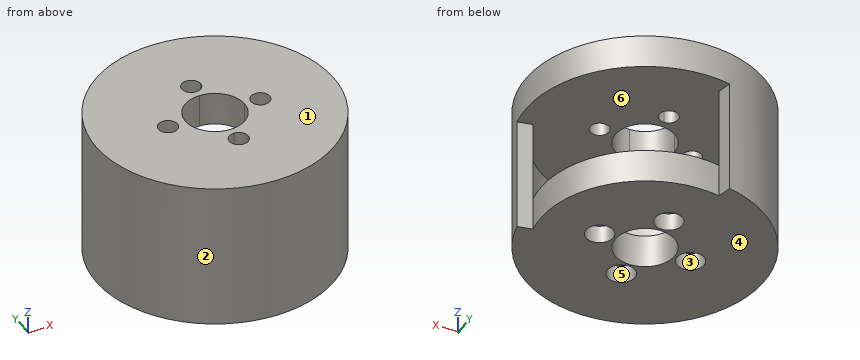
```python
from build123d import *

# Parameters (mm, degrees)
F0_R      = 25.4
F0_R_2    = 22.225
F0_R_3    = 6.35
F1_DEPTH  = 7.112
F2_R      = 25.4
F2_R_2    = 22.225
F3_DEPTH  = 17.272
F4_R      = 2.032
F5_DEPTH  = 21.29049
F6_R      = 2.921
F7_DEPTH  = 3.81
F9_DEPTH  = 17.272
F10_R     = 25.4
F10_R_2   = 2.032
F11_DEPTH = 7.112
F12_DEPTH = 25.4


with BuildPart() as f1:
    # F0 (on Top) → F1 (new body)
    with BuildSketch(Plane.XY):
        with Locations((-2.9115700163, -0.1164628848)):
            Circle(F0_R)
        with Locations((-2.9115700163, -0.1164628848)):
            Circle(F0_R_2, mode=Mode.SUBTRACT)
        with Locations((-2.9115700163, -0.1164628848)):
            Circle(F0_R_2)
        with Locations((-2.9115700163, -0.1164628848)):
            Circle(F0_R_3, mode=Mode.SUBTRACT)
    extrude(amount=F1_DEPTH)

    # F2 (on face) → F3 (join)
    with BuildSketch(Plane.XY.offset(7.112)):
        with Locations((-2.9115700163, -0.1164628848)):
            Circle(F2_R)
        with Locations((-2.9115700163, -0.1164628848)):
            Circle(F2_R_2, mode=Mode.SUBTRACT)
    extrude(amount=F3_DEPTH)

    # F4 (on face) → F5 (cut)
    with BuildSketch(Plane.XY.offset(7.112)):
        with Locations((-2.9115700163, 9.6625371152)):
            Circle(F4_R)
        with Locations((-12.6905700163, -0.1164628848)):
            Circle(F4_R)
        with Locations((6.8674299837, -0.1164628848)):
            Circle(F4_R)
        with Locations((-2.9115700163, -9.8954628848)):
            Circle(F4_R)
    extrude(amount=-F5_DEPTH, mode=Mode.SUBTRACT)

    # F6 (on face) → F7 (cut)
    with BuildSketch(Plane.XY):
        with Locations((-2.9112251941, -9.8947474398)):
            Circle(F6_R)
        with Locations((6.8677748059, -0.1157474398)):
            Circle(F6_R)
        with Locations((-2.9112251941, 9.6632525602)):
            Circle(F6_R)
        with Locations((-12.6902251941, -0.1157474398)):
            Circle(F6_R)
    extrude(amount=F7_DEPTH, mode=Mode.SUBTRACT)

    # F8 (on face) → F9 (cut)
    with BuildSketch(Plane.XY.offset(24.384)):
        with BuildLine():
            ThreePointArc((-7.4796047728, 21.634024086), (12.685813093, 15.5216009657), (18.8507418749, -4.6278269968))
            Line((18.8507418749, -4.6278269968), (21.9596435736, -5.2723075843))
            ThreePointArc((21.9596435736, -5.2723075843), (15.0679881207, 17.9099891283), (-8.1321811666, 24.7412365103))
            Line((-8.1321811666, 24.7412365103), (-7.4796047728, 21.634024086))
        make_face()
    extrude(amount=-F9_DEPTH, mode=Mode.SUBTRACT)

    # F10 (on face) → F11 (join)
    with BuildSketch(Plane.XY.offset(24.384)):
        with Locations((-2.9115700163, -0.1164628848)):
            Circle(F10_R)
        with BuildLine():
            ThreePointArc((-0.8795700163, -9.8954628848), (-4.3484109957, -11.3323038641), (-2.9115700163, -7.8634628848))
            ThreePointArc((-2.9115700163, -7.8634628848), (-1.4747290369, -8.4586219054), (-0.8795700163, -9.8954628848))
        make_face(mode=Mode.SUBTRACT)
        with Locations((-13.0211196663, -0.1164628848)):
            Circle(F10_R_2, mode=Mode.SUBTRACT)
        with BuildLine():
            ThreePointArc((-2.9115700163, 6.2335371152), (1.5785580442, 4.3736651758), (3.4384299837, -0.1164628848))
            ThreePointArc((3.4384299837, -0.1164628848), (1.5785580442, -4.6065909453), (-2.9115700163, -6.4664628848))
            ThreePointArc((-2.9115700163, -6.4664628848), (-7.4016980768, -4.6065909453), (-9.2615700163, -0.1164628848))
            ThreePointArc((-9.2615700163, -0.1164628848), (-7.4016980768, 4.3736651758), (-2.9115700163, 6.2335371152))
        make_face(mode=Mode.SUBTRACT)
        with BuildLine():
            ThreePointArc((8.8994299837, -0.1164628848), (6.8674299837, -2.1484628848), (4.8354299837, -0.1164628848))
            ThreePointArc((4.8354299837, -0.1164628848), (6.8674299837, 1.9155371152), (8.8994299837, -0.1164628848))
        make_face(mode=Mode.SUBTRACT)
        with BuildLine():
            ThreePointArc((-0.8795700163, 9.6625371152), (-1.4747290369, 8.2256961359), (-2.9115700163, 7.6305371152))
            ThreePointArc((-2.9115700163, 7.6305371152), (-4.3484109957, 11.0993780946), (-0.8795700163, 9.6625371152))
        make_face(mode=Mode.SUBTRACT)
    extrude(amount=F11_DEPTH)

    # F8 (on face) → F12 (cut)
    with BuildSketch(Plane.XY.offset(24.384)):
        with BuildLine():
            ThreePointArc((-7.4796047728, 21.634024086), (12.685813093, 15.5216009657), (18.8507418749, -4.6278269968))
            Line((18.8507418749, -4.6278269968), (21.9596435736, -5.2723075843))
            ThreePointArc((21.9596435736, -5.2723075843), (15.0679881207, 17.9099891283), (-8.1321811666, 24.7412365103))
            Line((-8.1321811666, 24.7412365103), (-7.4796047728, 21.634024086))
        make_face()
    extrude(amount=-F12_DEPTH, mode=Mode.SUBTRACT)


solid = f1.part
```
Read the model definition and answer for the solid it produces. Units are mm, in the model's axes. Face numbers are marked on the shaded views. A direction names the side the tool comes from. Give positions to 0.01 mm unless a question says otherwise; leave off trailing zeros. Order: outer loops, then holes, each group sorted by start corner. A loop starts at its lowest first (then second) coordinate and runs counter-clockwise, first axis right, second up.
(1) For a pull along X with two mould halves and no side action, classify the marked faces 1, 2 and 3 as released by +X, released by -X, zero draft, split by the parting line, or undercut.
(2) Find section C-C (x = 1). Give the vertices of the cut face in (y, z).
(3) Find section B-B (z = 29). Give the vertices of the cut face in (x, y).
(4) Given pin 1 (1.5 mm diameter, centred on x = -5.5, z = 21.5, fed in from -Y); pin 2 (5.5 mm diameter, centred on x = 6.87, y = -0.12, fed in from -Z); pin 3 (2 mm diameter, centred on y = 17.5, z = 25, fed in from +X), each flat-ended and moving along its own axis, determine where each tip first touches the part or whether it passes through.
(5) Find section A-A (y = 9). Give the vertices of the cut face in (x, z), plus the area to 3 significant figures.
(6) Straight lines are drawn through the part: L1, parallel to Z at x = 4, y = -14; L2, parallel to Y at x = -1.5, z = 28.5; L3, parallel to Y at x = -3.5, z = 22.5. For each, find the intervals that lie inside material, in ascending order.
(7) Find section D-D (y = -19.5). Give the vertices of the cut face in (x, z), plus the area to 3 significant figures.
(8) For the marked faces 4, 5 and 6, determine the directions among +Z, -Z, +X, -X, +Y, -Y from which every point of the face is accessible in a straight line to the end or side of a thin tool.
Result sheet:
1. face 1: zero draft
1. face 2: split by the parting line
1. face 3: undercut
2. outline: (-25.21, 0) - (-5.12, 0) - (-5.12, 7.11) - (-21.99, 7.11) - (-21.99, 24.38) - (-5.12, 24.38) - (-5.12, 31.5) - (-25.21, 31.5) - close; (4.89, 0) - (21.68, 0) - (21.68, 7.11) - (4.89, 7.11) - close; (4.89, 24.38) - (24.98, 24.38) - (24.98, 31.5) - (4.89, 31.5) - close
3. outline: circle Ø50.8 at (-2.91, -0.12); hole circle Ø4.06 at (-13.02, -0.12); hole circle Ø12.7 at (-2.91, -0.12); hole circle Ø4.06 at (-2.91, -9.9); hole circle Ø4.06 at (-2.91, 9.66); hole circle Ø4.06 at (6.87, -0.12)
4. pin 1: stops at y = -25.45
4. pin 2: stops at z = 3.81
4. pin 3: stops at x = 16.3
5. outline: (-26.62, 0) - (-5.76, 0) - (-5.76, 3.81) - (-4.83, 3.81) - (-4.83, 7.11) - (-23.18, 7.11) - (-23.18, 24.38) - (-4.83, 24.38) - (-4.83, 31.5) - (-26.62, 31.5) - close; (-0.99, 3.81) - (-0.07, 3.81) - (-0.07, 0) - (17.23, 0) - (17.23, 7.11) - (-0.99, 7.11) - close; (-0.99, 24.38) - (20.8, 24.38) - (20.8, 31.5) - (-0.99, 31.5) - close
5. area: 647 mm2
6. L1: z = 0 to 7.11, 24.38 to 31.5
6. L2: y = -25.48 to -11.36, -8.43 to -6.31, 6.07 to 8.2, 11.12 to 25.24
6. L3: y = -25.51 to -22.33
7. outline: (-19.33, 0) - (13.5, 0) - (13.5, 31.5) - (-19.33, 31.5) - close; hole (-13.78, 7.11) - (7.96, 7.11) - (7.96, 24.38) - (-13.78, 24.38) - close
7. area: 658 mm2
8. face 4: -Z, +X, -X, +Y, -Y
8. face 5: -Z
8. face 6: none
